```python
from build123d import *

# Parameters (mm, degrees)
SKETCH1_W               = 69.85
SKETCH1_H               = 69.85
BOSS_EXTRUDE1_DEPTH     = 4
SKETCH2_W               = 43.02
SKETCH2_H               = 43.02
SKETCH2_R               = 5.461
BOSS_EXTRUDE2_DEPTH     = 11
SKETCH3_R               = 5.461
CUT_EXTRUDE1_DEPTH      = 1
CUT_EXTRUDE1_DEPTH_BACK = 16
SKETCH4_W               = 43.02
SKETCH4_H               = 43.02
SKETCH4_W_2             = 9.122
SKETCH4_H_2             = 9.122
BOSS_EXTRUDE3_DEPTH     = 15


with BuildPart() as part:
    # Sketch1 → Boss-Extrude1 (new body)
    with BuildSketch(Plane(origin=(0, 0, 0), x_dir=(1, 0, 0), z_dir=(0, 1, 0))):
        with Locations((34.925, 34.925)):
            Rectangle(SKETCH1_W, SKETCH1_H)
    extrude(amount=BOSS_EXTRUDE1_DEPTH)

    # Sketch2 → Boss-Extrude2 (add)
    with BuildSketch(Plane(origin=(0, 4, 0), x_dir=(1, 0, 0), z_dir=(0, 1, 0))):
        with Locations((34.925, 34.925)):
            Rectangle(SKETCH2_W, SKETCH2_H)
        with Locations((23.876, 34.925)):
            Circle(SKETCH2_R, mode=Mode.SUBTRACT)
        with Locations((45.974, 34.925)):
            Circle(SKETCH2_R, mode=Mode.SUBTRACT)
    extrude(amount=BOSS_EXTRUDE2_DEPTH)

    # Sketch3 → Cut-Extrude1 (cut, two sides)
    with BuildSketch(Plane(origin=(0, 15, 0), x_dir=(1, 0, 0), z_dir=(0, 1, 0))) as cut_extrude1_sk:
        with Locations((23.876, 34.925)):
            Circle(SKETCH3_R)
        with Locations((45.974, 34.925)):
            Circle(SKETCH3_R)
    extrude(amount=CUT_EXTRUDE1_DEPTH, mode=Mode.SUBTRACT)
    extrude(cut_extrude1_sk.sketch, amount=-CUT_EXTRUDE1_DEPTH_BACK, mode=Mode.SUBTRACT)

    # Sketch4 → Boss-Extrude3 (add)
    with BuildSketch(Plane(origin=(0, 15, 0), x_dir=(1, 0, 0), z_dir=(0, 1, 0))):
        with Locations((34.925, 34.925)):
            Rectangle(SKETCH4_W, SKETCH4_H)
        with Locations((23.876, 34.925)):
            Rectangle(SKETCH4_W_2, SKETCH4_H_2, mode=Mode.SUBTRACT)
        with Locations((45.974, 34.925)):
            Rectangle(SKETCH4_W_2, SKETCH4_H_2, mode=Mode.SUBTRACT)
    extrude(amount=-BOSS_EXTRUDE3_DEPTH)


solid = part.part
```
For this review, take the finished solid that the model builds, in its own axes (mm). A direction names the side the tool comes from. Give positions to 0.01 mm unless a question says otherwise; leave off trailing zeros. Order: outer loops, then holes, each group sorted by start corner. A loop starts at its lowest first (then second) coordinate and runs counter-clockwise, first axis right, second up.
1) For faces 1 (the face through (56.435, 9, -35)), 2 (the face through (35, 9, -13.415)), 3 (the face through (50.535, 8, -35)), list the 3-axis set-ups (+Z, -Z, +X, -X, +Y, -Y) from which the entire face can be reached by the end or side of a thin tool; tool diameter is ignored.
2) Take a section at A-A (x = 46). Give the boundary of the cut face in (y, z) (3 decimals).
3) Wall thickness on line 1 (X direction, y = 1, z = -36.5) (3 decimals); line 2 (Z direction, x = 46, y = 14) (3 decimals); line 3 (Z direction, x = 49, y = 1): over which ranges is each line inside the solid? List them lowest first.
4) Take a section at C-C (z = -55). Give the boundary of the cut face in (x, y) (3 decimals), then the cut area to 3 significant figures.
5) Take a section at B-B (y = 6.75). Give the boundary of the cut face in (x, z) (3 decimals), then the cut area to 3 significant figures.
6) Insertion check: pin 1 (12 mm diameter, centred on x = 10.5, z = -30, fed in from +Y); pin 2 (5 mm diameter, centred on y = 9.5, z = -34, fed in from -X) (3 decimals); pin 3 (5 mm diameter, centred on x = 23, y = 8.5, fed in from +Z) (3 decimals); pin 4 (8 mm diameter, centred on x = 15, y = 11, fed in from -Z) (3 decimals). Each pin has a flat end and moves straight along its axis. Give the tip position at first contact, or say it passes through.
7) The part is to be moulded in two halves that separate along Z. For faces 4 (the face through (34, 2, 0)), 5 (the face through (46, 8, -39.486)), 6 (the face through (34, 0, -35)), say which applies: released by +Z, released by -Z, zero draft, split by the parting line, or undercut.
8) Take a section at D-D (x = 16.5). Give the boundary of the cut face in (y, z) (3 decimals), then the cut area to 3 significant figures.
Derived:
1. face 1: +Z, -Z, +X, +Y
1. face 2: +Z, +X, -X, +Y
1. face 3: +Y, -Y
2. outline: (0, -69.85) - (4, -69.85) - (4, -56.435) - (15, -56.435) - (15, -39.486) - (0, -39.486) - close; (0, -30.364) - (15, -30.364) - (15, -13.415) - (4, -13.415) - (4, 0) - (0, 0) - close
3. line 1: x = 0 to 19.315, 28.437 to 41.413, 50.535 to 69.85
3. line 2: z = -56.435 to -39.486, -30.364 to -13.415
3. line 3: z = -69.85 to -39.47, -30.38 to 0
4. outline: (0, 0) - (69.85, 0) - (69.85, 4) - (56.435, 4) - (56.435, 15) - (13.415, 15) - (13.415, 4) - (0, 4) - close
4. area: 753 mm2
5. outline: (13.415, -56.435) - (56.435, -56.435) - (56.435, -13.415) - (13.415, -13.415) - close; hole (19.315, -37.928) arc R5.461 ccw to (20.873, -39.486) - (26.879, -39.486) arc R5.461 ccw to (28.437, -37.928) - (28.437, -31.922) arc R5.461 ccw to (26.879, -30.364) - (20.873, -30.364) arc R5.461 ccw to (19.315, -31.922) - close; hole (41.413, -37.928) arc R5.461 ccw to (42.971, -39.486) - (48.977, -39.486) arc R5.461 ccw to (50.535, -37.928) - (50.535, -31.922) arc R5.461 ccw to (48.977, -30.364) - (42.971, -30.364) arc R5.461 ccw to (41.413, -31.922) - close
5. area: 1,690 mm2
6. pin 1: stops at y = 15
6. pin 2: stops at x = 13.415
6. pin 3: stops at z = -13.415
6. pin 4: stops at z = -56.435
7. face 4: released by +Z
7. face 5: undercut
7. face 6: zero draft
8. outline: (0, -69.85) - (4, -69.85) - (4, -56.435) - (15, -56.435) - (15, -13.415) - (4, -13.415) - (4, 0) - (0, 0) - close
8. area: 753 mm2
